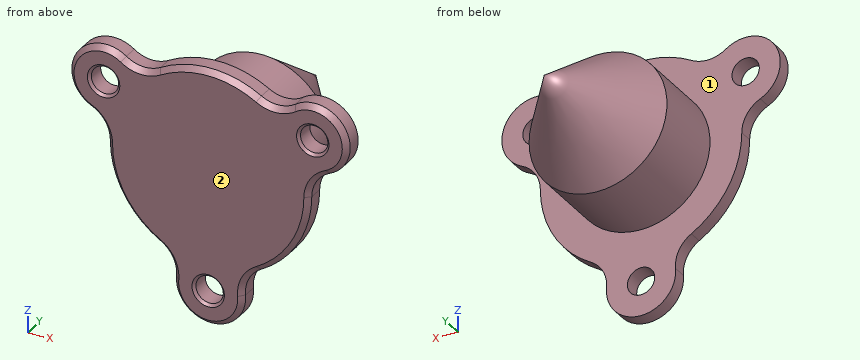
from build123d import *

# Parameters (mm, degrees)
SKETCH1_R           = 10.85
SKETCH1_R_2         = 2.15
BOSS_EXTRUDE1_DEPTH = 3
SKETCH1_2_R         = 10.85
BOSS_EXTRUDE2_DEPTH = 15
CHAMFER1_SIZE       = 0.8
CHAMFER2_SIZE       = 0.4


with BuildPart() as part:
    # Sketch1 → Boss-Extrude1 (new body)
    with BuildSketch(Plane(origin=(0, 0, 0), x_dir=(1, 0, 0), z_dir=(0, 1, 0))):
        with BuildLine():
            ThreePointArc((5.42820267, 18.513054646), (0, 24.45), (-5.42820267, 18.513054646))
            ThreePointArc((-5.42820267, 18.513054646), (-5.97168494, 15.760391094), (-7.912232668, 13.73386596))
            ThreePointArc((-7.912232668, 13.73386596), (-13.72650265, 7.925), (-15.849993148, -0.014738489))
            ThreePointArc((-15.849993148, -0.014738489), (-16.634741531, -2.708564686), (-18.74687696, -4.555565914))
            ThreePointArc((-18.74687696, -4.555565914), (-21.174321123, -12.225), (-13.31867429, -13.957488732))
            ThreePointArc((-13.31867429, -13.957488732), (-10.663056591, -13.051826408), (-7.937760479, -13.719127471))
            ThreePointArc((-7.937760479, -13.719127471), (0, -15.85), (7.937760479, -13.719127471))
            ThreePointArc((7.937760479, -13.719127471), (10.663056591, -13.051826408), (13.31867429, -13.957488732))
            ThreePointArc((13.31867429, -13.957488732), (21.174321123, -12.225), (18.74687696, -4.555565914))
            ThreePointArc((18.74687696, -4.555565914), (16.634741531, -2.708564686), (15.849993148, -0.014738489))
            ThreePointArc((15.849993148, -0.014738489), (13.72650265, 7.925), (7.912232668, 13.73386596))
            ThreePointArc((7.912232668, 13.73386596), (5.97168494, 15.760391094), (5.42820267, 18.513054646))
        make_face()
        Circle(SKETCH1_R, mode=Mode.SUBTRACT)
        with Locations((0, 19)):
            Circle(SKETCH1_R_2, mode=Mode.SUBTRACT)
        with Locations((16.454482672, -9.5)):
            Circle(SKETCH1_R_2, mode=Mode.SUBTRACT)
        with Locations((-16.454482672, -9.5)):
            Circle(SKETCH1_R_2, mode=Mode.SUBTRACT)
    extrude(amount=BOSS_EXTRUDE1_DEPTH)

    # Sketch1<2> → Boss-Extrude2 (add)
    with BuildSketch(Plane(origin=(0, 0, 0), x_dir=(1, 0, 0), z_dir=(0, 1, 0))):
        Circle(SKETCH1_2_R)
    extrude(amount=BOSS_EXTRUDE2_DEPTH)

    # Sketch2 → Revolve1 (revolve)
    with BuildSketch(Plane.XY):
        Polygon((0, 15), (10.85, 15), (0, 30), align=None)
    revolve(axis=Axis((0, 18.413549721, 0), (0, -1, 0)))

    # Chamfer1
    chamfer1_edges = [part.edges().sort_by_distance(p)[0] for p in [
        (16.634741531, 0, 2.708564686),
        (21.174321123, 0, 12.225),
        (10.663056591, 0, 13.051826408),
        (0, 0, 15.85),
        (-10.663056591, 0, 13.051826408),
        (-21.174321123, 0, 12.225),
        (-16.634741531, 0, 2.708564686),
        (-13.72650265, 0, -7.925),
        (-5.97168494, 0, -15.760391094),
        (0, 0, -24.45),
        (5.97168494, 0, -15.760391094),
        (13.72650265, 0, -7.925),
    ]]
    chamfer(chamfer1_edges, length=CHAMFER1_SIZE)

    # Chamfer2
    chamfer2_edges = [part.edges().sort_by_distance(p)[0] for p in [
        (-2.15, 0, -19),
        (14.304482672, 0, 9.5),
        (-18.604482672, 0, 9.5),
    ]]
    chamfer(chamfer2_edges, length=CHAMFER2_SIZE)


solid = part.part
Build history of the part. All positions in model axes, mm. Face numbers are marked on the shaded views. A direction names the side the tool comes from. Give positions to 0.01 mm unless a question says otherwise; leave off trailing zeros. Order: outer loops, then holes, each group sorted by start corner. A loop starts at its lowest first (then second) coordinate and runs counter-clockwise, first axis right, second up. Notation, with made-up numbers: M -19.5,-22 L -8.5,-22 A11 cw -8.5,-5 Z; hole C -38,2 d6. An arc over 180 degrees is marked long. Put each result on its own line as item: value.
Item 1: Cut at C-C on y = 24.25. Write the cut outline in (x, z), then the cut area to 3 significant figures.
Results are:
outline: C 0,0 d8.32
area: 54.3 mm2
Item 2: Cut at A-A on y = 6.25. Write the cut outline in (x, z), then the cut area to 3 significant figures.
Results are:
outline: C 0,0 d21.7
area: 370 mm2
Item 3: Drop flat-ended pins along their axis: pin 1 Ø6 at (x, y) = (2, 11) entering from -Z; pin 2 Ø6 at (y, z) = (14, -12) entering from +X; pin 3 Ø3 at (x, y) = (5.5, 17.5) entering from +Z. Give the stop position or say it passes through.
Results are:
pin 1: z = -10.85
pin 2: x = 6.06
pin 3: z = 8.78
Item 4: Wall check: probe 1 along X at (y, z) = (2.2, 9.5); probe 2 along Z at (x, y) = (0, 1.4); probe 3 along X at (y, z) = (1.25, -19). Give the ranges that are in metal, low to high.
Results are:
probe 1: -21.9 to -18.6, -14.3 to 14.3, 18.6 to 21.9
probe 2: -24.45 to -21.15, -16.85 to 15.85
probe 3: -5.45 to -2.15, 2.15 to 5.45
Item 5: Cut at B-B on z = 9.5. Count the separate pieces of the cut face and the enclosed holes in it, then the cut area to 3 significant figures.
Results are:
separate pieces: 3
enclosed holes: 0
area: 243 mm2
Item 6: Which spindle directions (+Z, -Z, +X, -X, +Y, -Y) get a long thin tool onto all of the face, cutting with end or side? Do the marked faces 1 and 2. Say none if no direction does.
Results are:
face 1: +Y
face 2: +Z, -Z, +X, -X, -Y
